from build123d import *

# Parameters (mm, degrees)
SKETCH1_W           = 96
SKETCH1_H           = 66
SKETCH1_R           = 2
BOSS_EXTRUDE1_DEPTH = 2
SKETCH8_R           = 2.375
BOSS_EXTRUDE3_DEPTH = 7.5
SKETCH9_R           = 2.55
CUT_EXTRUDE1_DEPTH  = 7.5


with BuildPart() as part:
    # Sketch1 → Boss-Extrude1 (new body)
    with BuildSketch(Plane(origin=(0, 0, 0), x_dir=(1, 0, 0), z_dir=(0, 1, 0))):
        with Locations((48, 33)):
            Rectangle(SKETCH1_W, SKETCH1_H)
        with Locations(Location((33, 33, 0), (0, 0, 270))):
            Circle(SKETCH1_R, mode=Mode.SUBTRACT)
        with Locations(Location((63, 33, 0), (0, 0, 270))):
            Circle(SKETCH1_R, mode=Mode.SUBTRACT)
    extrude(amount=BOSS_EXTRUDE1_DEPTH)

    # Sketch8 → Boss-Extrude3 (add)
    with BuildSketch(Plane.ZY.offset(-27)):
        with BuildLine():
            Line((-8.517353084, 0), (0, 0))
            ThreePointArc((0, 0), (-12.462971529, -9.886825426), (-27.6351276, -14.670198345))
            ThreePointArc((-27.6351276, -14.670198345), (-33, -20.375), (-38.3648724, -14.670198345))
            ThreePointArc((-38.3648724, -14.670198345), (-53.537028471, -9.886825426), (-66, 0))
            Line((-66, 0), (-57.482646916, 0))
            ThreePointArc((-57.482646916, 0), (-33, -9), (-8.517353084, 0))
        make_face()
        with Locations((-33, -15)):
            Circle(SKETCH8_R, mode=Mode.SUBTRACT)
    boss_extrude3 = extrude(amount=BOSS_EXTRUDE3_DEPTH)

    # Mirror1: Boss-Extrude3 across plane
    add(boss_extrude3.mirror(Plane.ZY.offset(-48)))

    # Sketch9 → Cut-Extrude1 (cut)
    with BuildSketch(Plane(origin=(76.5, 0, 0), x_dir=(0, 0, -1), z_dir=(1, 0, 0))):
        with Locations((33, -15)):
            Circle(SKETCH9_R)
    extrude(amount=-CUT_EXTRUDE1_DEPTH, mode=Mode.SUBTRACT)


solid = part.part
Input: part model. Units: mm. Frame: model coordinates. A direction names the side the tool comes from. Coordinates: 2 decimals unless noted, no trailing zeros. Order: outer loops, then holes, each group sorted by start corner. A loop starts at its lowest first (then second) coordinate and runs counter-clockwise, first axis right, second up. Notation, with made-up numbers: M 41,44 L 78,44 A14 ccw 78,71 Z; hole C 44,30 d8. An arc over 180 degrees is marked long. Write item = value, one per line. Start each with the question number.
(1) Reachability of faces 1 (the flat face through (27, -11, -33)), 2 (the flat face through (76.5, -9.4, -32.8)), 3 (the cylindrical face through (72.802, -14.888, -30.452)), 4 (the flat face through (47, 2, -33)), 5 (the flat face through (47, 1, -66)) from +Z, -Z, +X, -X, +Y, -Y: full face, straight path, thin tool, end or side. Return the list, or none.
(2) Section B-B on z = -33. Output: boundary loops of the cut face in (x, y) (3 decimals).
(3) First-contact query: P1, Ø12, axis at x = 62, y = -14, coming from the -Z side; P2, Ø6.5, axis at x = 63, z = -33, coming from the +Y side; P3, Ø6, axis at y = -15, z = -33, coming from the +X side; P4, Ø12, axis at y = -12.5, z = -31.5, coming from the -X side. Flat tips, straight axial feed; report the tip coordinate or a pass-through.
(4) Section A-A on x = 33. Output: boundary loops of the cut face in (y, z).
(5) Line query: line 1 along Y through (x, z) = (73, -33) (3 decimals); line 2 along X through (y, z) = (0.55, -33); line 3 along Y through (x, z) = (38.5, -50). Output: solid intervals per line, ascending. Write a range as [from, to].
(6) Pull-direction query (Z, two-part tool) for faces 6 (the flat face through (47, 1, 0)), 7 (the cylindrical face through (23.3, -16.45, -34.88)), 8 (the flat face through (69, -9.4, -32.8)), 9 (the cylindrical face through (64.686, 0.986, -31.925)); classes: released by +Z, released by -Z, zero draft, split by the parting line, or undercut.
(7) Section D-D on y = -7.25. Output: boundary loops of the cut face in (x, z), and give its area (3 significant figures).
(8) Section C-C on z = -41. Output: boundary loops of the cut face in (x, y).
Result set:
q1.face_1 = +Z, -Z, -Y
q1.face_2 = +Z, -Z, +X, -Y
q1.face_3 = +X
q1.face_4 = +Z, -Z, +X, -X, +Y
q1.face_5 = -Z, +X, -X, +Y, -Y
q2.outline = M 0,0 L 31,0 L 31,2 L 0,2 Z; M 19.5,-20.375 L 27,-20.375 L 27,-17.375 L 19.5,-17.375 Z; M 19.5,-12.625 L 27,-12.625 L 27,-9 L 19.5,-9 Z; M 35,0 L 61,0 L 61,2 L 35,2 Z; M 65,0 L 96,0 L 96,2 L 65,2 Z; M 69,-20.375 L 76.5,-20.375 L 76.5,-17.55 L 69,-17.55 Z; M 69,-12.45 L 76.5,-12.45 L 76.5,-9 L 69,-9 Z
q3.P1 = through
q3.P2 = 2
q3.P3 = 76.5
q3.P4 = 19.5
q4.outline = M 0,-66 L 2,-66 L 2,-35 L 0,-35 Z; M 0,-31 L 2,-31 L 2,0 L 0,0 Z
q5.line_1 = [-20.375, -17.55], [-12.45, -9], [0, 2]
q5.line_2 = [0, 31], [35, 61], [65, 96]
q5.line_3 = [0, 2]
q6.face_6 = released by +Z
q6.face_7 = undercut
q6.face_8 = zero draft
q6.face_9 = undercut
q7.outline = M 19.5,-57.88 L 27,-57.88 L 27,-44.37 L 19.5,-44.37 Z; M 19.5,-21.63 L 27,-21.63 L 27,-8.12 L 19.5,-8.12 Z; M 69,-57.88 L 76.5,-57.88 L 76.5,-44.37 L 69,-44.37 Z; M 69,-21.63 L 76.5,-21.63 L 76.5,-8.12 L 69,-8.12 Z
q7.area = 405 mm²
q8.outline = M 0,0 L 96,0 L 96,2 L 0,2 Z; M 19.5,-14.26 L 27,-14.26 L 27,-8.14 L 19.5,-8.14 Z; M 69,-14.26 L 76.5,-14.26 L 76.5,-8.14 L 69,-8.14 Z
